CAD build for the part. Positions are in the model's coordinates, mm. A direction names the side the tool comes from. Round coordinates to 2 decimals unless told otherwise and drop trailing zeros. Loops run counter-clockwise (first coordinate to the right, second up) from the corner with the lowest first, then second, coordinate; pieces in that order, holes last.
```python
from build123d import *

# Parameters (mm, degrees)
SWEEP1_PROFILE_R                           = 5
SKETCH17_R                                 = 3.5
CUT_EXTRUDE1_DEPTH                         = 55.313902456
SKETCH18_W                                 = 31.905055519
SKETCH18_H                                 = 6.394424732
CUT_EXTRUDE2_DEPTH                         = 7
MIRROR1_AT_THE_SECOND_PLANE_COPY_1_SKETC_W = 31.905055519
MIRROR1_AT_THE_SECOND_PLANE_COPY_1_SKETC_H = 6.394424732
MIRROR1_AT_THE_SECOND_PLANE_COPY_1_DEPTH   = 7


with BuildPart() as part:
    # Sweep1: sweep along a path in Sketch1
    with BuildLine(Plane.XY) as sweep1_path:
        Line((-25, 0), (-25, -40))
        Line((-25, -40), (0, -40))
        Line((0, -40), (25, -40))
        Line((25, -40), (25, 0))
    # Sweep1 profile (on start of the path) → Sweep1 (sweep)
    with BuildSketch(Plane(origin=(-25, 0, 0), x_dir=(0, 0, -1), z_dir=(0, -1, 0))):
        Circle(SWEEP1_PROFILE_R)
    sweep(path=sweep1_path.line, transition=Transition.RIGHT)

    # Sketch17 → Cut-Extrude1 (cut, through all)
    with BuildSketch(Plane(origin=(0, 0, 0), x_dir=(1, 0, 0), z_dir=(0, 1, 0))):
        with Locations(Location((-25, 0, 0), (0, 0, 180))):
            Circle(SKETCH17_R)
        with Locations(Location((25, 0, 0), (0, 0, 180))):
            Circle(SKETCH17_R)
    extrude(amount=-CUT_EXTRUDE1_DEPTH, mode=Mode.SUBTRACT)

    # Sketch18 → Cut-Extrude2 (cut)
    with BuildSketch(Plane(origin=(-8.964466094, 0, -8.964466094), x_dir=(0, 1, 0), z_dir=(0.7071067811865488, 0, 0.7071067811865464))):
        with Locations((-18.731085844, 17.249970265)):
            Rectangle(SKETCH18_W, SKETCH18_H)
    cut_extrude2 = extrude(amount=-CUT_EXTRUDE2_DEPTH, mode=Mode.SUBTRACT)

    # Mirror1: Cut-Extrude2 across plane
    add(cut_extrude2.mirror(Plane(origin=(-8.964466094, 0, -8.964466094), x_dir=(-0.7071067811865465, 0, 0.7071067811865486), z_dir=(0.7071067811865488, 0, 0.7071067811865464))), mode=Mode.SUBTRACT)

    # Mirror1 at the second plane: Cut-Extrude2 across plane
    add(cut_extrude2.mirror(Plane(origin=(0, 0, 0), x_dir=(0, 0, 1), z_dir=(1, 0, 0))), mode=Mode.SUBTRACT)

    # Mirror1 at the second plane copy 1 sketc → Mirror1 at the second plane copy 1 (cut)
    with BuildSketch(Plane(origin=(8.964466094, 0, -8.964466094), x_dir=(0, 1, 0), z_dir=(0.707106781186549, 0, -0.7071067811865466))):
        with Locations((-18.731085844, 17.249970265)):
            Rectangle(MIRROR1_AT_THE_SECOND_PLANE_COPY_1_SKETC_W, MIRROR1_AT_THE_SECOND_PLANE_COPY_1_SKETC_H)
    extrude(amount=-MIRROR1_AT_THE_SECOND_PLANE_COPY_1_DEPTH, mode=Mode.SUBTRACT)


solid = part.part
```
Item 1: Cut at B-B, the plane y = -40. Give the cut face in (x, z).
Answers follow:
outline: (-25, -5) - (25, -5) arc R5 ccw to (25, 5) - (-25, 5) arc R5 ccw to start; hole circle Ø7 at (-25, 0); hole circle Ø7 at (25, 0)
Item 2: Cut at D-D, the plane x = 3.5. Give the cut face in (y, z).
Answers follow:
outline: circle Ø10 at (-40, 0)
Item 3: Cut at C-C, the plane z = 2. Give the cut face in (x, y), plus the area to 3 significant figures.
Answers follow:
outline: (-29.58, -44.58) - (-27.87, -44.58) - (-27.87, 0) - (-29.58, 0) - close; (-22.13, -44.58) - (22.13, -44.58) - (22.13, -34.68) - (20.42, -34.68) - (20.42, -35.42) - (-20.42, -35.42) - (-20.42, -34.68) - (-22.13, -34.68) - close; (-22.13, -2.78) - (-20.42, -2.78) - (-20.42, 0) - (-22.13, 0) - close; (20.42, -2.78) - (22.13, -2.78) - (22.13, 0) - (20.42, 0) - close; (27.87, -44.58) - (29.58, -44.58) - (29.58, 0) - (27.87, 0) - close
area: 570 mm2
Item 4: Two-plate mould, pull along Z, no slides. Class faces 1 (the flat face through (-21.899, -18.954, -2.026)), 2 (the flat face through (22.8, 0, 3.3)), 3 (the flat face through (-24.72, -18.954, 4.197)), 4 (the cylindrical face through (0.42, -44.88, 1.08)): released by +Z, released by -Z, zero draft, split by the parting line, or undercut.
Answers follow:
face 1: released by +Z
face 2: zero draft
face 3: undercut
face 4: split by the parting line
Item 5: Flat gauge pins, fed straight in: P1, Ø3, axis at x = 19.5, y = -24.5, coming from the +Z side; P2, Ø1.5, axis at x = 0, y = -39, coming from the -Z side. Where does each tip first touch, or does it go through?
Answers follow:
P1: stops at z = -0.13
P2: stops at z = -4.99
Item 6: 3-axis set-ups, long thin cutter, end or side, ignore diameter. For faces 5 (the cylindrical face through (-28.34, -22.19, 1.05)), 6 (the flat face through (21.899, -18.954, -2.026)), 7 (the cylindrical face through (-29.436, -22.815, -2.307)), 8 (the flat face through (24.72, -18.954, 4.197)), 9 (the flat face through (-27.2, 0, -3.3)): which of +Z, -Z, +X, -X, +Y, -Y reach the whole face in a straight line?
Answers follow:
face 5: +Y, -Y
face 6: +Z
face 7: +Y
face 8: none
face 9: +Z, -Z, +X, -X, +Y
Item 7: Probe line 1 (X direction, y = -36, z = 0); line 2 (X direction, y = -33, z = 0); line 3 (X direction, y = -38, z = -1.25). List the from-to ranges inside material, lowest first.
Answers follow:
line 1: x = -30 to -28.5, -21.5 to 21.5, 28.5 to 30
line 2: x = -30 to -28.5, 28.5 to 30
line 3: x = -29.84 to -28.27, -21.73 to 21.73, 28.27 to 29.84
